```python
from build123d import *

# Parameters (mm, degrees)
SKETCH1_R               = 50.8
BOSS_EXTRUDE1_DEPTH     = 107.95
SKETCH2_R               = 38.1
BOSS_EXTRUDE2_DEPTH     = 6.35
BOSS_EXTRUDE3_START     = 69.85
SKETCH3_R               = 38.1
BOSS_EXTRUDE3_DEPTH     = 69.85
SKETCH4_R               = 30.48
BOSS_EXTRUDE4_DEPTH     = 10.16
SKETCH5_R               = 15.875
CUT_EXTRUDE1_DEPTH      = 82.55
SKETCH7_OUTSIDE_W       = 151.932
SKETCH7_OUTSIDE_H       = 151.932
SKETCH7_OUTSIDE_W_2     = 98.552
SKETCH7_OUTSIDE_H_2     = 127
CUT_EXTRUDE2_DEPTH      = 107.95
F_1_2_20_TAPPED_HOLE1_D = 11.50874
F_1_4_20_TAPPED_HOLE1_D = 5.1054


with BuildPart() as part:
    # Sketch1 → Boss-Extrude1 (new body)
    with BuildSketch(Plane(origin=(0, 0, 0), x_dir=(1, 0, 0), z_dir=(0, 1, 0))):
        with Locations(Location((0, 0, 0), (0, 0, 270))):
            Circle(SKETCH1_R)
    extrude(amount=BOSS_EXTRUDE1_DEPTH)

    # Sketch2 → Boss-Extrude2 (add)
    with BuildSketch(Plane(origin=(0, 107.95, 0), x_dir=(1, 0, 0), z_dir=(0, 1, 0))):
        with Locations(Location((0, 0, 0), (0, 0, 270))):
            Circle(SKETCH2_R)
    extrude(amount=BOSS_EXTRUDE2_DEPTH)

    # Sketch3 → Boss-Extrude3 (add)
    with BuildSketch(Plane.XZ.offset(BOSS_EXTRUDE3_START)):
        with Locations(Location((0, 0, 0), (0, 0, 90))):
            Circle(SKETCH3_R)
    extrude(amount=-BOSS_EXTRUDE3_DEPTH)

    # Sketch4 → Boss-Extrude4 (add)
    with BuildSketch(Plane.XZ.offset(69.85)):
        with Locations(Location((0, 0, 0), (0, 0, 270))):
            Circle(SKETCH4_R)
    extrude(amount=BOSS_EXTRUDE4_DEPTH)

    # Sketch5 → Cut-Extrude1 (cut)
    with BuildSketch(Plane.XZ.offset(80.01)):
        with Locations(Location((0, 0, 0), (0, 0, 270))):
            Circle(SKETCH5_R)
    extrude(amount=-CUT_EXTRUDE1_DEPTH, mode=Mode.SUBTRACT)

    # Sketch7 outside → Cut-Extrude2 (cut)
    with BuildSketch(Plane(origin=(0, 107.95, 0), x_dir=(1, 0, 0), z_dir=(0, 1, 0))):
        Rectangle(SKETCH7_OUTSIDE_W, SKETCH7_OUTSIDE_H)
        Rectangle(SKETCH7_OUTSIDE_W_2, SKETCH7_OUTSIDE_H_2, mode=Mode.SUBTRACT)
    extrude(amount=-CUT_EXTRUDE2_DEPTH, mode=Mode.SUBTRACT)

    # 1/2-20 Tapped Hole1 (through all)
    with Locations(Plane.ZY.offset(49.276)):
        with Locations((0, 53.975)):
            Hole(F_1_2_20_TAPPED_HOLE1_D / 2)

    # 1/4-20 Tapped Hole1 (through all)
    with Locations(Plane.ZY.offset(49.276)):
        with Locations((0, 85.725), (0, 22.225)):
            Hole(F_1_4_20_TAPPED_HOLE1_D / 2)


solid = part.part
```
Check sheet for the modelled part. Datum: model origin and axes. Units: mm. A direction names the side the tool comes from. Round coordinates to 2 decimals unless told otherwise and drop trailing zeros. Order: outer loops, then holes, each group sorted by start corner. A loop starts at its lowest first (then second) coordinate and runs counter-clockwise, first axis right, second up. Notation, with made-up numbers: M 73.5,62.5 L 113.5,62.5 A14 ccw 113.5,86.5 Z; hole C 69,68 d8. An arc over 180 degrees is marked long. Answer in a Markdown table with one row per item.
(1) Gauge pin test, flat ends, axial feed: pin 1 (1.5 mm diameter, centred on x = 18, z = 39, fed in from +Y); pin 2 (2 mm diameter, centred on y = -35, z = 29.5, fed in from -X); pin 3 (12 mm diameter, centred on y = 13, z = -21.5, fed in from +X). Record the tip position at first contact, or that the pin passes through.
Findings:
| item | result |
|---|---|
| pin 1 | stops at y = 107.95 |
| pin 2 | stops at x = -25.29 |
| pin 3 | stops at x = 48.38 |
(2) Set-up check for faces 5 (the flat face through (1, 114.3, -1)), 6 (the flat face through (-26, -69.85, -17)), 7 (the cylindrical face through (-23.183, 111.081, -30.235)): record each of +Z, -Z, +X, -X, +Y, -Y from which the full face is reachable in a straight line by a thin tool's end or side.
Findings:
| item | result |
|---|---|
| face 5 | +Z, -Z, +X, -X, +Y |
| face 6 | -Y |
| face 7 | +Y |
(3) Section check A-A on z = 0. Give the number of separate pieces and of enclosed holes in the cut face, plus the area to 3 significant figures.
Findings:
| item | result |
|---|---|
| separate pieces | 4 |
| enclosed holes | 0 |
| area | 12,300 mm^2 |
(4) Material ranges on line 1 along Y through (x, z) = (-25, 0); line 2 along Y through (x, z) = (12.5, 0); line 3 along Y through (x, z) = (-17, -39), recorded low to high. Write a range as from..to.
Findings:
| item | result |
|---|---|
| line 1 | y = -80.01..19.67, 24.78..48.22, 59.73..83.17, 88.28..114.3 |
| line 2 | y = 2.54..19.67, 24.78..48.22, 59.73..83.17, 88.28..114.3 |
| line 3 | y = 0..107.95 |
(5) Section check D-D on z = 25. Record the boundary of the cut face in (x, y), plus the area to 3 significant figures.
Findings:
| item | result |
|---|---|
| outline | M -44.22,0 L -28.75,0 L -28.75,-69.85 L -17.44,-69.85 L -17.44,-80.01 L 17.44,-80.01 L 17.44,-69.85 L 28.75,-69.85 L 28.75,0 L 44.22,0 L 44.22,107.95 L 28.75,107.95 L 28.75,114.3 L -28.75,114.3 L -28.75,107.95 L -44.22,107.95 Z |
| area | 14,300 mm^2 |
(6) Section check C-C on y = -4.5. Record the boundary of the cut face in (x, z) (3 decimals), plus the area to 3 significant figures.
Findings:
| item | result |
|---|---|
| outline | C 0,0 d76.2; hole C 0,0 d31.75 |
| area | 3,770 mm^2 |
(7) Section check B-B on x = -26.5. Record the boundary of the cut face in (y, z) (3 decimals).
Findings:
| item | result |
|---|---|
| outline | M -80.01,-15.059 L -69.85,-15.059 L -69.85,-27.374 L 0,-27.374 L 0,-43.34 L 107.95,-43.34 L 107.95,-27.374 L 114.3,-27.374 L 114.3,27.374 L 107.95,27.374 L 107.95,43.34 L 0,43.34 L 0,27.374 L -69.85,27.374 L -69.85,15.059 L -80.01,15.059 Z; hole C 22.225,0 d5.105; hole C 53.975,0 d11.509; hole C 85.725,0 d5.105 |
(8) Draft check along Z on faces 1 (the cylindrical face through (0.69, 20.672, 2.026)), 2 (the cylindrical face through (23.183, -35.414, -30.235)), 3 (the flat face through (-32, 107.95, 22)), 4 (the cylindrical face through (0.94, 53.22, -50.79)). Enter one of: +Z half, -Z half, draft (parallel to the pull), parting line (faces both ways), or undercut.
Findings:
| item | result |
|---|---|
| face 1 | undercut |
| face 2 | parting line |
| face 3 | draft |
| face 4 | -Z half |
